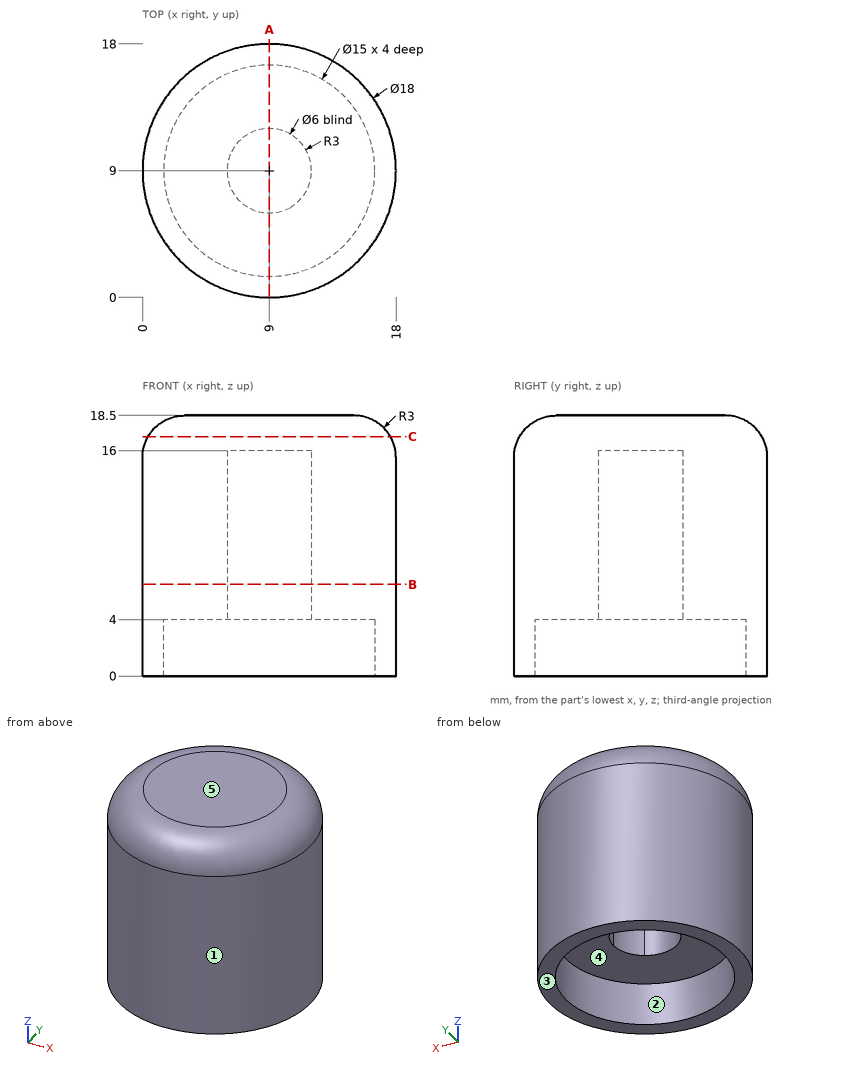
Drawing for the job (mm, zero at the part's lowest x, y, z). A direction names the side the tool comes from. Round coordinates to 2 decimals unless told otherwise and drop trailing zeros. Write each loop counter-clockwise with the first axis right and the second up, starting at its lowest first coordinate (ties: lowest second). Pieces come first, ordered by that corner, then holes. Notation, with made-up numbers: M 27.5,10 L 49.5,10 A22 cw 49.5,19 Z; hole C -10.5,13.5 d2. An arc over 180 degrees is marked long. Answer as a JSON object with one key per item and string values. Group by question number.
(1) Mould opens along X. For the marked faces 1, 2 and 3 say: pulls with the +X half, pulls with the -X half, needs draft (parallel to the pull), parting line crosses it, or undercut.
(2) Drill centre lines: L1, parallel to Y at x = 9, z = 10; L2, parallel to Z at x = 13, y = 5.75; L3, parallel to Y at x = 10, z = 4.75. Where is each one in solid material? Low to high.
(3) Cut at C-C (z = 17). Give the cut face in (x, y), and give its area (3 significant figures).
(4) Which spindle directions (+Z, -Z, +X, -X, +Y, -Y) get a long thin tool onto all of the face, cutting with end or side? Do the marked faces 4 and 5. Say none if no direction does.
(5) Cut at B-B (z = 6.5). Give the cut face in (x, y).
(6) Cut at A-A (x = 9). Give the cut face in (y, z).
(7) Flat gauge pins, fed straight in: pin 1 (6 mm diameter, centred on x = 12.5, z = 15.5, fed in from +Y); pin 2 (1 mm diameter, centred on y = 3.5, z = 10, fed in from -X); pin 3 (1 mm diameter, centred on y = 14.5, z = 10, fed in from +X). Where does each tip first touch, or does it go through?
Responses:
{
 "1": {"face 1": "parting line crosses it", "face 2": "undercut", "face 3": "needs draft"},
 "2": {"L1": "y = 0 to 6, 12 to 18", "L2": "z = 4 to 18.5", "L3": "y = 0.06 to 6.17, 11.83 to 17.94"},
 "3": {"outline": "C 9,9 d17.2", "area": "232 mm2"},
 "4": {"face 4": "-Z", "face 5": "+Z, +X, -X, +Y, -Y"},
 "5": {"outline": "C 9,9 d18; hole C 9,9 d6"},
 "6": {"outline": "M 0,0 L 1.5,0 L 1.5,4 L 6,4 L 6,16 L 12,16 L 12,4 L 16.5,4 L 16.5,0 L 18,0 L 18,15.5 A3 ccw 15,18.5 L 3,18.5 A3 ccw 0,15.5 Z"},
 "7": {"pin 1": "stops at y = 17.99", "pin 2": "stops at x = 1.52", "pin 3": "stops at x = 16.48"}
}
